Design review of the part built by this model. Coordinates are the model's own, in mm. A direction names the side the tool comes from. Give positions to 0.01 mm unless a question says otherwise; leave off trailing zeros. Order: outer loops, then holes, each group sorted by start corner. A loop starts at its lowest first (then second) coordinate and runs counter-clockwise, first axis right, second up. Notation, with made-up numbers: (-22.75, 70.5) -> (7.25, 70.5) arc R24 cw to (7.25, 107.5) -> close; hole circle Ø2 at (32, -31). An arc over 180 degrees is marked (long way). Answer in a Markdown table with one row per item. Add a question column.
Autodesk Inventor part; units mm, degrees
ref_plane "Plano de trabalho1" through (0, -25, 0) normal (0, 1, 0) x (-1, 0, 0)
ref_plane "Plano de trabalho2" through (0, 0, 62.5) normal (0, 0, 1) x (1, 0, 0)
ref_plane "YZ Plane" through (0, 0, 0) normal (1, 0, 0) x (0, 1, 0)
sketch "Esboço1" plane through (0, 0, 0) normal (0, 0, 1) x (1, 0, 0)
  arc A0 (5.7143, 49.6724) -> (5.7143, -49.6724) centre (0, 0) ccw
  arc A1 (178.4286, -29.8034) -> (178.4286, 29.8034) centre (175, 0) ccw
  line L0 (5.7143, 49.6724) -> (178.4286, 29.8034)
  line L1 (0, 0) -> (175, 0) construction
  line L2 (5.7143, -49.6724) -> (178.4286, -29.8034)
  circle A2 centre (0, 0) radius 32.5
  circle A3 centre (175, 0) radius 12.5
  point P0 (-54.0476, 56.5474)
  point P1 (215.9085, 25.4918)
  point P2 (-54.0476, -56.5474)
  point P3 (215.9085, -25.4918)
  dimension "d0" = 100
  dimension "d1" = 60
  dimension "d2" = 175
  dimension "d3" = 65
  dimension "d4" = 25
extrude "Extrusão1" add sketch "Esboço1" along normal blind 125
ref_plane "Plano de trabalho1" through (0, -25, 0) normal (0, 1, 0) x (-1, 0, 0)
sketch "Esboço2" plane through (0, -25, 0) normal (0, 1, 0) x (-1, 0, 0)
  line L0 (0, 0) -> (0, 125) construction
  line L1 (50, 125) -> (-5.7143, 125) construction
  line L2 (0, 62.5) -> (109.1848, 62.5) construction
  circle A0 centre (75, 62.5) radius 25
  dimension "d8" = 50
  dimension "d9" = 75
extrude "Extrusão2" add sketch "Esboço2" along normal blind 80
sketch "Esboço3" plane through (0, -25, 0) normal (0, 1, 0) x (-1, 0, 0)
  circle A0 centre (75, 62.5) radius 25
  arc A1 (83.5505, 85.9923) -> (83.5505, 39.0077) centre (75, 62.5) ccw
  line L0 (83.5505, 39.0077) -> (39.6496, 23.0291)
  line L1 (50, 125) -> (-5.7143, 125)
  line L2 (75, 62.5) -> (-32.0182, 62.5) construction
  line L3 (83.5505, 85.9923) -> (39.6496, 101.9709)
  line L4 (39.6496, 23.0291) -> (39.6496, 101.9709)
  point P0 (0, 0)
  point P1 (94.387, 42.9518)
  point P2 (9.9213, 12.2089)
  point P3 (94.387, 82.0482)
  point P4 (9.9213, 112.7911)
  point P5 (83.5505, 39.0077)
  dimension "d12" = 20
extrude "Extrusão3" add sketch "Esboço3" along normal blind 50 contours A0 L0 L4 L3
ref_plane "Plano de trabalho2" through (0, 0, 62.5) normal (0, 0, 1) x (1, 0, 0)
sketch "Esboço4" plane through (0, 0, 62.5) normal (0, 0, 1) x (1, 0, 0)
  line L0 (-50, 55) -> (-100, 55)
  line L1 (-75, 37.5468) -> (-75, 0)
  arc A0 (-8.6824, 49.2404) -> (-50, 0) centre (0, 0) ccw
  line L2 (-75, 0) -> (-50, 0)
  line L3 (-75, 37.5468) -> (-8.6824, 49.2404)
  dimension "d16" = 100
  dimension "d17" = 80
extrude "Extrusão4" add sketch "Esboço4" along normal mid plane 15
sketch "Esboço5" plane through (0, 0, 0) normal (0, 1, 0) x (-1, 0, 0)
  line L0 (0, 0) -> (0, 125) construction
  line L1 (0, 62.5) -> (-205, 62.5) construction
  line L2 (-205, 0) -> (-205, 125) construction
  arc A0 (-80, 25) -> (-80, 100) centre (-80, 62.5) ccw
  line L3 (-80, 25) -> (-214.9719, 25)
  line L4 (-80, 100) -> (-214.9719, 100)
  line L5 (-214.9719, 100) -> (-214.9719, 25)
  dimension "d20" = 75
  dimension "d21" = 80
extrude "Extrusão5" cut sketch "Esboço5" against normal through all both and the other way through all
sketch "Esboço6" plane through (-75, 55, 62.5) normal (0, 1, 0) x (1, 0, 0)
  point P0 (75, 62.5)
  point P1 (0, 0)
  point P2 (0, 0)
hole "Furo1" at (-75, 55, 62.5) at (-75, 55, 62.5) direction (0, -1, 0) diameter 25 end through all counterbore diameter 30 counterbore depth 8
sketch "Esboço7" plane through (0, 0, 125) normal (0, 0, 1) x (1, 0, 0)
  circle A0 centre (175, 0) radius 12.5
  circle A1 centre (175, 0) radius 15
  point P0 (0, 0)
  dimension "d31" = 30
extrude "Extrusão6" cut sketch "Esboço7" against normal blind 2.5
sketch "Esboço8" plane through (0, 0, 0) normal (0, 0, -1) x (-1, 0, 0)
  circle A0 centre (-175, 0) radius 12.5
  circle A1 centre (-175, 0) radius 15
  point P0 (0, 0)
  dimension "d34" = 30
extrude "Extrusão7" cut sketch "Esboço8" against normal blind 2.5
properties part number "Rubia_ASR3"
1) For L1, parallel to X at y = 4.5, z = 71; L2, parallel to X at y = 51.75, z = 62.5; L3, parallel to Z at x = 95.5, y = 10, list the stretches that pass through material, from the lowest coordinate up.
2) Add section B-B, the plane z = 62.5. Write out the cut boundary in (x, y).
3) Mouldability with a two-part tool opening along Y and no side actions: class faces 5 (the face through (-54, 25, 86)), 6 (the face through (171.6, 12.3, 122.5)), 7 (the face through (-35.804, -34.901, 61.625)), 8 (the face through (186.923, -3.755, 111.092)) as +Y half, -Y half, draft (parallel to the pull), parting line (faces both ways), or undercut.
4) Clearance check with a flat-ended pin moving along its axis: P1, Ø15, axis at x = 178.5, y = -5.5, coming from the -Z side. State where the tip first meets the part, or that it passes through.
5) Add section A-A, the plane x = 0. Write out the cut boundary in (y, z), and give its area (4 significant figures).
6) Add section C-C, the plane y = 0. Give the number of separate pieces and of enclosed holes in the cut face, and give its area (3 significant figures).
7) Machinability: for faces 1 (the face through (-39, 37, 70)), 2 (the face through (178.4, 12.3, 2.5)), 3 (the face through (-54, 25, 40)), 4 (the face through (-98.09, 23.33, 72.08)), which of the approach directions +Z, -Z, +X, -X, +Y, -Y give a long, thin tool a straight path to every point of the face, cutting with its end or side? Answer none if there is none.
8) Add section D-D, the plane x = 175. Write out the cut boundary in (y, z), and give its area (3 significant figures).
Verdict:
| question | item | result |
|---|---|---|
| 1 | L1 | x = -98.51 to -84.17, -65.83 to -32.19, 32.19 to 43.48 |
| 1 | L2 | x = -100 to -90, -60 to -50 |
| 1 | L3 | z = 0 to 25, 100 to 125 |
| 2 | outline | (-100, -25) -> (-87.5, -25) -> (-87.5, 47) -> (-90, 47) -> (-90, 55) -> (-100, 55) -> close; (-62.5, -25) -> (-43.3, -25) arc R50 ccw to (5.71, -49.67) -> (42.5, -45.44) -> (42.5, 45.44) -> (5.71, 49.67) arc R50 ccw to (-8.68, 49.24) -> (-50, 41.95) -> (-50, 55) -> (-60, 55) -> (-60, 47) -> (-62.5, 47) -> close; hole circle Ø65 at (0, 0) |
| 3 | face 5 | +Y half |
| 3 | face 6 | undercut |
| 3 | face 7 | parting line |
| 3 | face 8 | undercut |
| 4 | P1 | stops at z = 2.5 |
| 5 | outline | (-50, 0) -> (-32.5, 0) -> (-32.5, 125) -> (-50, 125) -> close; (32.5, 0) -> (50, 0) -> (50, 125) -> (32.5, 125) -> close |
| 5 | area | 4,375 mm2 |
| 6 | separate pieces | 4 |
| 6 | enclosed holes | 1 |
| 6 | area | 12,900 mm2 |
| 7 | face 1 | +Z, +Y |
| 7 | face 2 | -Z |
| 7 | face 3 | -Z, +Y |
| 7 | face 4 | +Y |
| 8 | outline | (-30.2, 0) -> (-15, 0) -> (-15, 2.5) -> (-12.5, 2.5) -> (-12.5, 25) -> (-30.2, 25) -> close; (-30.2, 100) -> (-12.5, 100) -> (-12.5, 122.5) -> (-15, 122.5) -> (-15, 125) -> (-30.2, 125) -> close; (12.5, 2.5) -> (15, 2.5) -> (15, 0) -> (30.2, 0) -> (30.2, 25) -> (12.5, 25) -> close; (12.5, 100) -> (30.2, 100) -> (30.2, 125) -> (15, 125) -> (15, 122.5) -> (12.5, 122.5) -> close |
| 8 | area | 1,740 mm2 |
